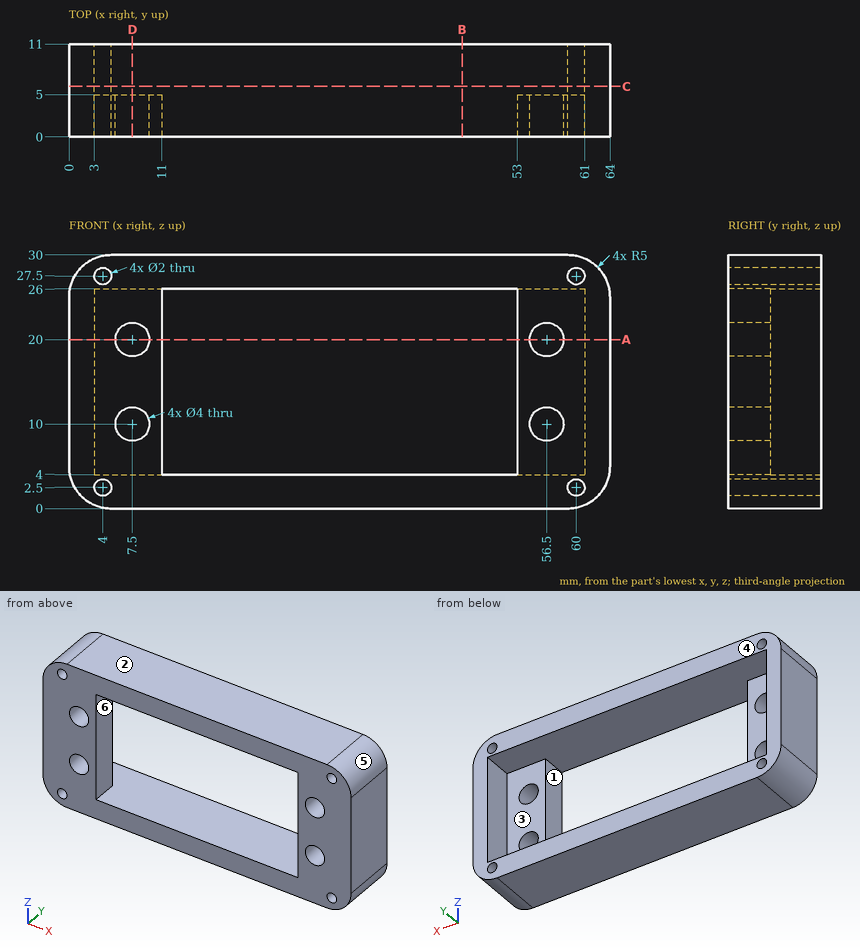
The figure shows three views and two pictorial views of one solid part (mm, origin at its lowest corner). Answer the questions. A direction names the side the tool comes from. Round coordinates to 2 decimals unless told otherwise and drop trailing zeros. Order: outer loops, then holes, each group sorted by start corner. A loop starts at its lowest first (then second) coordinate and runs counter-clockwise, first axis right, second up. Notation, with made-up numbers: M -9.75,28.5 L 29.25,28.5 A27 ccw 29.25,57.5 Z; hole C -34.75,20.5 d11. An arc over 180 degrees is marked long. Answer in a Markdown table with one row per item. Add a question column.
1) The part is cut by section B-B on x = 46.5. Determine the outline of the cut face in (y, z), plus the area to 3 significant figures.
2) Determine the mould class of the marked faces 4, 5 and 6 for opening direction Z: pulls with the +Z half, pulls with the -Z half, needs draft (parallel to the pull), parting line crosses it, or undercut.
3) The part is cut by section A-A on z = 20. Determine the outline of the cut face in (x, y), plus the area to 3 significant figures.
4) Flat-ended cylindrical pins translate along their axes: pin 1 Ø6 at (x, z) = (27, 22.5) entering from +Y; pin 2 Ø2.5 at (x, z) = (58.5, 15.5) entering from +Y; pin 3 Ø3 at (x, z) = (60, 2.5) entering from -Y; pin 4 Ø1.5 at (y, z) = (7.5, 3.5) entering from +X. Find the tip coordinate at first contact, or state that the pin passes through.
5) Consider line 1 along X through (y, z) = (1.55, 20); line 2 along X through (y, z) = (0.5, 7.5); line 3 along X through (y, z) = (4.75, 10.75). Determine where each line is inside the solid, lowest interval first. Write a range as from..to.
6) Which of the six approach directions +Z, -Z, +X, -X, +Y, -Y give full straight-line access (tool end or side, diameter ignored) to the marked faces 1, 2 and 3?
7) The part is cut by section C-C on y = 6. Determine the outline of the cut face in (x, z), plus the area to 3 significant figures.
8) The part is cut by section D-D on x = 7.5. Determine the outline of the cut face in (y, z).
Findings below:
| question | item | result |
|---|---|---|
| 1 | outline | M 0,0 L 11,0 L 11,4 L 0,4 Z; M 0,26 L 11,26 L 11,30 L 0,30 Z |
| 1 | area | 88.0 mm² |
| 2 | face 4 | needs draft |
| 2 | face 5 | pulls with the +Z half |
| 2 | face 6 | undercut |
| 3 | outline | M 0,0 L 5.5,0 L 5.5,5 L 3,5 L 3,11 L 0,11 Z; M 9.5,0 L 11,0 L 11,5 L 9.5,5 Z; M 53,0 L 54.5,0 L 54.5,5 L 53,5 Z; M 58.5,0 L 64,0 L 64,11 L 61,11 L 61,5 L 58.5,5 Z |
| 3 | area | 106 mm² |
| 4 | pin 1 | passes through |
| 4 | pin 2 | stops at y = 5 |
| 4 | pin 3 | stops at y = 0 |
| 4 | pin 4 | stops at x = 63.94 |
| 5 | line 1 | x = 0..5.5, 9.5..11, 53..54.5, 58.5..64 |
| 5 | line 2 | x = 0..11, 53..64 |
| 5 | line 3 | x = 0..5.65, 9.35..11, 53..54.65, 58.35..64 |
| 6 | face 1 | +Y, -Y |
| 6 | face 2 | +Z, +X, -X, +Y, -Y |
| 6 | face 3 | +Y |
| 7 | outline | M 0,5 A5 ccw 5,0 L 59,0 A5 ccw 64,5 L 64,25 A5 ccw 59,30 L 5,30 A5 ccw 0,25 Z; hole C 4,2.5 d2; hole M 3,4 L 61,4 L 61,26 L 3,26 Z; hole C 4,27.5 d2; hole C 60,2.5 d2; hole C 60,27.5 d2 |
| 7 | area | 610 mm² |
| 8 | outline | M 0,0 L 11,0 L 11,4 L 5,4 L 5,8 L 0,8 Z; M 0,12 L 5,12 L 5,18 L 0,18 Z; M 0,22 L 5,22 L 5,26 L 11,26 L 11,30 L 0,30 Z |
